from build123d import *

# Parameters (mm, degrees)
SKETCH_1_R               = 12.5
SKETCH_1_R_2             = 3
EXTRUDE_1_DEPTH          = 3
HOLE_WIZARD_M3_2_D       = 2.5
CUT_EXTRUDE_1_DEPTH      = 19.668154703
CUT_EXTRUDE_1_DEPTH_BACK = 19.668154703
HOLE_WIZARD_M3_1_D       = 2.5
CHAMFER_1_SIZE           = 0.5


with BuildPart() as part:
    # 草图1 → 凸台-拉伸1 (new, symmetric)
    with BuildSketch(Plane(origin=(0, 0, 0), x_dir=(1, 0, 0), z_dir=(0, 1, 0))):
        with Locations(Location((0, 0, 0), (0, 0, 270))):
            Circle(SKETCH_1_R)
        with Locations(Location((0, 0, 0), (0, 0, 270))):
            Circle(SKETCH_1_R_2, mode=Mode.SUBTRACT)
    extrude(amount=EXTRUDE_1_DEPTH, both=True)

    # M3 螺纹孔2 (through all)
    with Locations(Plane(origin=(0, 3, -10), x_dir=(0, 0, 1), z_dir=(0, 1, 0))):
        with Locations((0, 0), (10, 10), (20, 0), (10, -10)):
            Hole(HOLE_WIZARD_M3_2_D / 2)

    # 草图4 → 切除-拉伸1 (cut, two sides: drawn at the far end of the back side and taken through both)
    with BuildSketch(Plane(origin=(0, 3, 0), x_dir=(1, 0, 0), z_dir=(0, 1, 0)).offset(-CUT_EXTRUDE_1_DEPTH_BACK)):
        Polygon((-79.861969102, -2), (-12.338962679, -2), (12.338962679, -2), (79.861969102, -2), (79.861969102, -137.046012846), (-79.861969102, -137.046012846), align=None)
    extrude(amount=CUT_EXTRUDE_1_DEPTH + CUT_EXTRUDE_1_DEPTH_BACK, mode=Mode.SUBTRACT)

    # M3 螺纹孔1 (through all)
    with Locations(Plane(origin=(-5.5, 0, 2), x_dir=(1, 0, 0), z_dir=(0, 0, 1))):
        with Locations((0, 0), (11, 0)):
            Hole(HOLE_WIZARD_M3_1_D / 2)

    # 倒角1
    chamfer_1_edges = [part.edges().sort_by_distance(p)[0] for p in [
        (0, -3, -3),
        (0, 3, -3),
    ]]
    chamfer(chamfer_1_edges, length=CHAMFER_1_SIZE)


solid = part.part
Work out the finished part from the listing and answer in its coordinate system (mm). Give positions to 0.01 mm unless a question says otherwise; leave off trailing zeros. Loops run counter-clockwise (first coordinate to the right, second up) from the corner with the lowest first, then second, coordinate; pieces in that order, holes last. Notation, with made-up numbers: (38.25, 32.5) -> (44.25, 32.5) arc R20 ccw to (44.25, 60.5) -> close; hole circle Ø8 at (-11, -20). An arc over 180 degrees is marked (long way). Use a Markdown table: item, result. Add a question column.
1. Flat-ended cylindrical pins translate along their axes: pin 1 Ø1.5 at (y, z) = (2.5, -3) entering from -X; pin 2 Ø4 at (x, z) = (0, -10) entering from -Y; pin 3 Ø3 at (y, z) = (-1, -9) entering from -X; pin 4 Ø3 at (y, z) = (-0.5, -10) entering from -X. Find the tip coordinate at first contact, or state that the pin passes through.
2. Section D-D on y = -2 is taken. Determine the outline of the cut face in (x, z).
3. Find the intervals of material crossed by probe 1 along X at (y, z) = (-1.5, -2); probe 2 along X at (y, z) = (0, -7.75); probe 3 along X at (y, z) = (-1, -1.75), in increasing order.
4. Section B-B on x = -10 is taken. Determine the outline of the cut face in (y, z), and give its area (3 significant figures).
5. Section A-A on z = -10 is taken. Determine the outline of the cut face in (x, y), and give its area (3 significant figures).
6. Section C-C on z = 0 is taken. Determine the outline of the cut face in (x, y), and give its area (3 significant figures).
7. Determine the mould class of faces 1 (the cylindrical face through (0.303, 0.042, -12.496)), 2 (the cylindrical face through (0, 0, -3)), 3 (the flat face through (0, -3, -5)) for opening direction X: released by +X, released by -X, zero draft, split by the parting line, or undercut.
Results below:
| question | item | result |
|---|---|---|
| 1 | pin 1 | stops at x = -12.3 |
| 1 | pin 2 | stops at y = -3 |
| 1 | pin 3 | stops at x = -10 |
| 1 | pin 4 | stops at x = -9.17 |
| 2 | outline | (-12.34, 2) arc R12.5 ccw (long way) to (12.34, 2) -> (2.24, 2) arc R3 cw (long way) to (-2.24, 2) -> close; hole circle Ø2.5 at (-10, 0); hole circle Ø2.5 at (0, -10); hole circle Ø2.5 at (10, 0) |
| 3 | probe 1 | x = -12.34 to -2.24, 2.24 to 12.34 |
| 3 | probe 2 | x = -9.81 to -6.75, -4.25 to 4.25, 6.75 to 9.81 |
| 3 | probe 3 | x = -12.38 to -6.25, -4.75 to -2.44, 2.44 to 4.75, 6.25 to 12.38 |
| 4 | outline | (-3, -7.5) -> (3, -7.5) -> (3, -1.25) -> (-3, -1.25) -> close; (-3, 1.25) -> (3, 1.25) -> (3, 2) -> (-3, 2) -> close |
| 4 | area | 42.0 mm^2 |
| 5 | outline | (-7.5, -3) -> (-1.25, -3) -> (-1.25, 3) -> (-7.5, 3) -> close; (1.25, -3) -> (7.5, -3) -> (7.5, 3) -> (1.25, 3) -> close; hole circle Ø2.5 at (-5.5, 0); hole circle Ø2.5 at (5.5, 0) |
| 5 | area | 65.2 mm^2 |
| 6 | outline | (-12.5, -3) -> (-11.25, -3) -> (-11.25, 3) -> (-12.5, 3) -> close; (-8.75, -3) -> (-3.5, -3) -> (-3, -2.5) -> (-3, 2.5) -> (-3.5, 3) -> (-8.75, 3) -> close; (3, -2.5) -> (3.5, -3) -> (8.75, -3) -> (8.75, 3) -> (3.5, 3) -> (3, 2.5) -> close; (11.25, -3) -> (12.5, -3) -> (12.5, 3) -> (11.25, 3) -> close; hole circle Ø2.5 at (-5.5, 0); hole circle Ø2.5 at (5.5, 0) |
| 6 | area | 73.7 mm^2 |
| 7 | face 1 | split by the parting line |
| 7 | face 2 | undercut |
| 7 | face 3 | zero draft |
